Could you check a few things on this model? Use its own coordinates, in mm. A direction names the side the tool comes from. Round coordinates to 2 decimals unless told otherwise and drop trailing zeros. Loops run counter-clockwise (first coordinate to the right, second up) from the corner with the lowest first, then second, coordinate; pieces in that order, holes last. Notation, with made-up numbers: M 19.25,3 L 39.25,3 A33 cw 39.25,40 Z; hole C 46,19 d4. An arc over 180 degrees is marked long. One line per item, written item: value. Start each with the question number.
Q1. Imagine slicing it at A-A (y = 5). Please give me the cut outline in (x, z), then the cut area to 3 significant figures.
Q2. Thinking about a two-plate mould opening in X: for faces 1 (the face through (24, 6, 0)), 2 (the face through (-24, 6, 0)), 3 (the face through (-10.74, -18.07, -2.38)), which applies, released by +X, released by -X, zero draft, split by the parting line, or undercut?
Q3. Imagine slicing it at B-B (x = 0). Please give me the cut outline in (y, z).
Q4. I'm going to push flat-ended pins straight in: pin 1 Ø3 at (y, z) = (-33.5, 10) entering from +X; pin 2 Ø5 at (x, y) = (0, -18) entering from -Z; pin 3 Ø3 at (y, z) = (-27.5, 9) entering from -X. Where does each tip first touch, or does it pass through?
Q5. Which directions (+Z, -Z, +X, -X, +Y, -Y) give clear straight access to the entire face, cutting with the end or side of a thin tool? Please do faces 4 (the face through (-21.43, 6.08, -0.65)), 5 (the face through (11, 0, -9)).
Q6. Imagine slicing it at C-C (z = 7.5). Please give me the cut outline in (x, y), then the cut area to 3 significant figures.
Q7. Imagine slicing it at D-D (z = 0). Please give me the cut outline in (x, y).
Q8. Please list where these lines run through material, in increasing order: line 1 along X through (y, z) = (-26.5, -0.5); line 2 along Y through (x, z) = (13, 18); line 3 along Z through (x, y) = (-9, -30).
from build123d import *

# Parameters (mm, degrees)
BOSS_EXTRUDE1_DEPTH = 12
SKETCH2_R           = 14
BOSS_EXTRUDE2_DEPTH = 49
SKETCH3_R           = 11
SKETCH3_R_2         = 3
CUT_EXTRUDE1_DEPTH  = 69.534662763


with BuildPart() as part:
    # Sketch1 → Boss-Extrude1 (new body)
    with BuildSketch(Plane(origin=(0, 0, 0), x_dir=(1, 0, 0), z_dir=(0, 1, 0))):
        with BuildLine():
            Line((0, 20), (13.266499161, 20))
            ThreePointArc((13.266499161, 20), (24, 0), (13.266499161, -20))
            Line((13.266499161, -20), (-13.266499161, -20))
            ThreePointArc((-13.266499161, -20), (-24, 0), (-13.266499161, 20))
            Line((-13.266499161, 20), (0, 20))
        make_face()
    extrude(amount=BOSS_EXTRUDE1_DEPTH)

    # Sketch2 → Boss-Extrude2 (add)
    with BuildSketch(Plane.XZ):
        with Locations(Location((0, 0, 0), (0, 0, 90))):
            Circle(SKETCH2_R)
    extrude(amount=BOSS_EXTRUDE2_DEPTH)

    # Sketch3 → Cut-Extrude1 (cut, through all)
    with BuildSketch(Plane(origin=(0, 12, 0), x_dir=(1, 0, 0), z_dir=(0, 1, 0))):
        with Locations(Location((0, 0, 0), (0, 0, 270))):
            Circle(SKETCH3_R)
        with Locations(Location((-11.5, 14.491376746, 0), (0, 0, 270))):
            Circle(SKETCH3_R_2)
        with Locations(Location((-18.5, 0, 0), (0, 0, 270))):
            Circle(SKETCH3_R_2)
        with Locations(Location((-11.5, -14.491376746, 0), (0, 0, 270))):
            Circle(SKETCH3_R_2)
        with Locations(Location((11.5, -14.491376746, 0), (0, 0, 270))):
            Circle(SKETCH3_R_2)
        with Locations(Location((18.5, 0, 0), (0, 0, 270))):
            Circle(SKETCH3_R_2)
        with Locations(Location((11.5, 14.491376746, 0), (0, 0, 270))):
            Circle(SKETCH3_R_2)
    extrude(amount=-CUT_EXTRUDE1_DEPTH, mode=Mode.SUBTRACT)


solid = part.part
Report:
1. outline: M -13.27,-20 L 13.27,-20 A24 ccw 13.27,20 L -13.27,20 A24 ccw Z; hole C -18.5,0 d6; hole C -11.5,-14.49 d6; hole C -11.5,14.49 d6; hole C 0,0 d22; hole C 11.5,-14.49 d6; hole C 11.5,14.49 d6; hole C 18.5,0 d6
1. area: 1,120 mm²
2. face 1: released by +X
2. face 2: released by -X
2. face 3: undercut
3. outline: M -49,-14 L 0,-14 L 0,-20 L 12,-20 L 12,-11 L -49,-11 Z; M -49,11 L 12,11 L 12,20 L 0,20 L 0,14 L -49,14 Z
4. pin 1: stops at x = 11.12
4. pin 2: stops at z = -14
4. pin 3: stops at x = -11.82
5. face 4: +Y, -Y
5. face 5: -Y
6. outline: M -22.8,0 L -11.82,0 L -11.82,-49 L -8.05,-49 L -8.05,12 L -22.8,12 Z; M 8.05,-49 L 11.82,-49 L 11.82,0 L 22.8,0 L 22.8,12 L 8.05,12 Z
6. area: 724 mm²
7. outline: M -24,0 L -21.5,0 L -21.5,12 L -24,12 Z; M -15.5,0 L -14,0 L -14,-49 L -11,-49 L -11,12 L -15.5,12 Z; M 11,-49 L 14,-49 L 14,0 L 15.5,0 L 15.5,12 L 11,12 Z; M 21.5,0 L 24,0 L 24,12 L 21.5,12 Z
8. line 1: x = -13.99 to -10.99, 10.99 to 13.99
8. line 2: y = 0 to 12
8. line 3: z = -10.72 to -6.32, 6.32 to 10.72
